Check sheet for the modelled part. Datum: model origin and axes. Units: mm. A direction names the side the tool comes from. Coordinates: 2 decimals unless noted, no trailing zeros. Loops run counter-clockwise (first coordinate to the right, second up) from the corner with the lowest first, then second, coordinate; pieces in that order, holes last. Notation, with made-up numbers: (8.5, 15.5) - (13.5, 15.5) arc R21 ccw to (13.5, 24.5) - close; hole circle Ø11 at (4, -10.75). An arc over 180 degrees is marked (long way). Use a Markdown table: item, result. Add a question column.
1) Tool access check on faces 4 (the flat face through (100, 2, 1)), 5 (the flat face through (-1, 4, -64)). Record the directions out of +Z, -Z, +X, -X, +Y, -Y that give a thin tool (end or side, any length) a straight path to the whole face; none if there is none.
2) Sectioned sample at C-C, the plane y = -7. Enter the section's corners in (x, z), then the cut area to 3 significant figures.
3) Thickness scan on line 1 (X direction, y = 2.5, z = 32.5); line 2 (Z direction, x = -52.5, y = 0.5); line 3 (Y direction, x = 28, z = -39). Record the ranges inside material, lowest first.
4) Draft check along X on faces 1 (the flat face through (104, 4, 1)), 2 (the flat face through (-100, 2, 1)), 3 (the flat face through (-90, -16, -50)). Enter one of: pulls with the +X half, pulls with the -X half, needs draft (parallel to the pull), parting line crosses it, or undercut.
5) Go/stop test with flat-tipped pins: P1, Ø10, axis at x = -25.5, z = 51, coming from the -Y side; P2, Ø10, axis at y = -8, z = -9.5, coming from the -X side. Record where each tip stops, or that it passes through.
6) Sectioned sample at B-B, the plane z = 50. Enter the section's corners in (x, y).
7) Sectioned sample at A-A, the plane x = -58. Enter the section's corners in (y, z).
8) Sectioned sample at D-D, the plane x = 90. Enter the section's corners in (y, z), then the cut area to 3 significant figures.
from build123d import *

# Parameters (mm, degrees)
CROQUIS1_W              = 208
CROQUIS1_H              = 128
SALIENTE_EXTRUIR1_DEPTH = 8
CROQUIS1_4_W            = 200
CROQUIS1_4_H            = 120
CORTAR_EXTRUIR1_DEPTH   = 4
CROQUIS2_R              = 2.5
SALIENTE_EXTRUIR2_DEPTH = 20


with BuildPart() as part:
    # Croquis1 → Saliente-Extruir1 (new body)
    with BuildSketch(Plane(origin=(0, 0, 0), x_dir=(1, 0, 0), z_dir=(0, 1, 0))):
        Rectangle(CROQUIS1_W, CROQUIS1_H)
    extrude(amount=SALIENTE_EXTRUIR1_DEPTH)

    # Croquis1<4> → Cortar-Extruir1 (cut)
    with BuildSketch(Plane(origin=(0, 0, 0), x_dir=(1, 0, 0), z_dir=(0, 1, 0))):
        Rectangle(CROQUIS1_4_W, CROQUIS1_4_H)
    extrude(amount=CORTAR_EXTRUIR1_DEPTH, mode=Mode.SUBTRACT)

    # Croquis2 → Saliente-Extruir2 (add)
    with BuildSketch(Plane.XZ.offset(-4)):
        with Locations((-90, -50)):
            Circle(CROQUIS2_R)
        with Locations((90, 50)):
            Circle(CROQUIS2_R)
    extrude(amount=SALIENTE_EXTRUIR2_DEPTH)


solid = part.part
Solved:
| question | item | result |
|---|---|---|
| 1 | face 4 | -Y |
| 1 | face 5 | -Z, +X, -X, +Y, -Y |
| 2 | outline | circle Ø5 at (-90, -50); circle Ø5 at (90, 50) |
| 2 | area | 39.3 mm2 |
| 3 | line 1 | x = -104 to -100, 100 to 104 |
| 3 | line 2 | z = -64 to -60, 60 to 64 |
| 3 | line 3 | y = 4 to 8 |
| 4 | face 1 | pulls with the +X half |
| 4 | face 2 | undercut |
| 4 | face 3 | needs draft |
| 5 | P1 | stops at y = 4 |
| 5 | P2 | passes through |
| 6 | outline | (-104, 0) - (-100, 0) - (-100, 4) - (87.5, 4) - (87.5, -16) - (92.5, -16) - (92.5, 4) - (100, 4) - (100, 0) - (104, 0) - (104, 8) - (-104, 8) - close |
| 7 | outline | (0, -64) - (8, -64) - (8, 64) - (0, 64) - (0, 60) - (4, 60) - (4, -60) - (0, -60) - close |
| 8 | outline | (-16, 47.5) - (4, 47.5) - (4, -60) - (0, -60) - (0, -64) - (8, -64) - (8, 64) - (0, 64) - (0, 60) - (4, 60) - (4, 52.5) - (-16, 52.5) - close |
| 8 | area | 644 mm2 |
